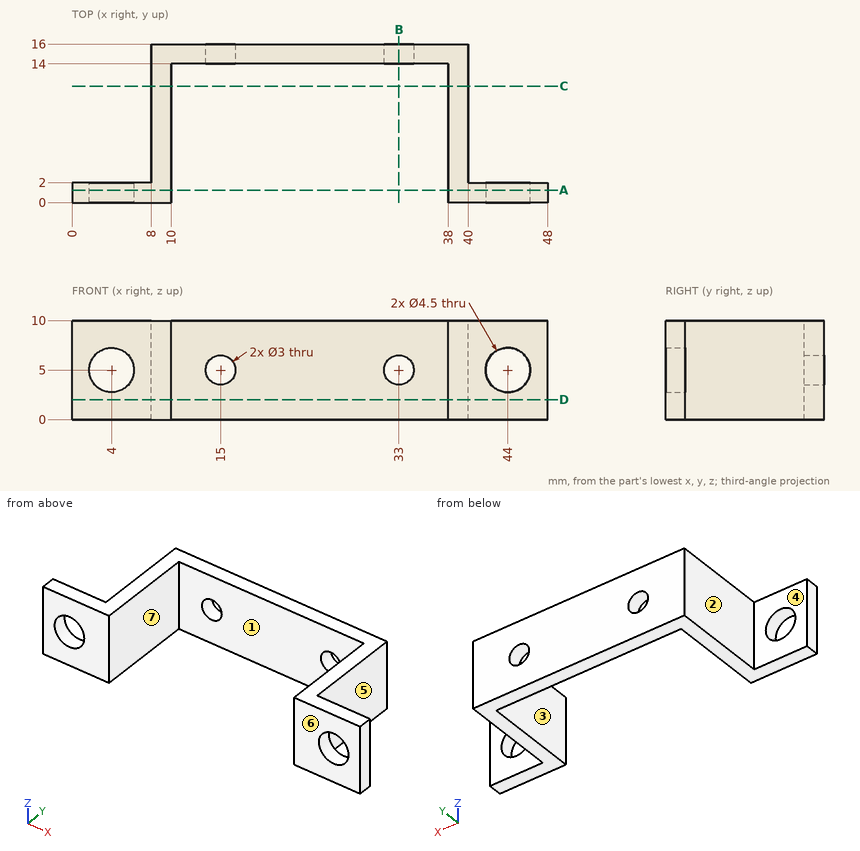
The drawing under review shows one solid part. Ordinate dimensions are in mm from its lowest x, y, z. A direction names the side the tool comes from. Coordinates: 2 decimals unless noted, no trailing zeros. Order: outer loops, then holes, each group sorted by start corner. A loop starts at its lowest first (then second) coordinate and runs counter-clockwise, first axis right, second up. Notation, with made-up numbers: (83, -27) -> (136, -27) arc R16 cw to (136, -23) -> close; hole circle Ø11 at (86, -18). An arc over 180 degrees is marked (long way). Return JSON: item names as keys, results as strings.
1. For line 1 (X direction, y = 0.7, z = 5); line 2 (X direction, y = 14.7, z = 5); line 3 (Z direction, x = 15, y = 14.45), list the stretches that pass through material, from the lowest coordinate up. Write a range as from..to.
Answer block:
{"line 1": "0..1.75, 6.25..10, 38..41.75, 46.25..48", "line 2": "8..13.5, 16.5..31.5, 34.5..40", "line 3": "0..3.5, 6.5..10"}
2. Machinability: for the marked faces 5, 6 and 7, which of the approach directions +Z, -Z, +X, -X, +Y, -Y give a long, thin tool a straight path to every point of the face, cutting with its end or side? Answer none if there is none.
Answer block:
{"face 5": "+Z, -Z, +X, +Y", "face 6": "+Z, -Z, +X, -X, -Y", "face 7": "+Z, -Z, -Y"}
3. We need section B-B on x = 33. Write out the cut boundary in (y, z), and give its area (3 significant figures).
Answer block:
{"outline": "(14, 0) -> (16, 0) -> (16, 3.5) -> (14, 3.5) -> close; (14, 6.5) -> (16, 6.5) -> (16, 10) -> (14, 10) -> close", "area": "14.0 mm²"}
4. We need section D-D on z = 2. Write out the cut boundary in (x, y).
Answer block:
{"outline": "(0, 0) -> (10, 0) -> (10, 14) -> (38, 14) -> (38, 0) -> (48, 0) -> (48, 2) -> (40, 2) -> (40, 16) -> (8, 16) -> (8, 2) -> (0, 2) -> close"}
5. We need section C-C on y = 11.75. Write out the cut boundary in (x, z), and give its area (3 significant figures).
Answer block:
{"outline": "(8, 0) -> (10, 0) -> (10, 10) -> (8, 10) -> close; (38, 0) -> (40, 0) -> (40, 10) -> (38, 10) -> close", "area": "40.0 mm²"}
6. We need section A-A on y = 1.25. Write out the cut boundary in (x, z).
Answer block:
{"outline": "(0, 0) -> (10, 0) -> (10, 10) -> (0, 10) -> close; (38, 0) -> (48, 0) -> (48, 10) -> (38, 10) -> close; hole circle Ø4.5 at (4, 5); hole circle Ø4.5 at (44, 5)"}
7. The part is to be moulded in two halves that separate along X. For the marked faces 1, 2, 3 and 4, say which applies: +X half, -X half, draft (parallel to the pull), parting line (faces both ways), or undercut.
Answer block:
{"face 1": "undercut", "face 2": "-X half", "face 3": "undercut", "face 4": "draft"}
8. For pin 1 Ø2.5 at (x, z) = (33, 5) entering from +Y; pin 2 Ø2.5 at (x, z) = (44.5, 7.5) entering from +Y; pin 3 Ø3 at (y, z) = (7, 4.5) entering from -X; pin 4 Ø3 at (y, z) = (5, 6.5) entering from +X, all flat-tipped, find the tip position at first contact; note any pin that passes through.
Answer block:
{"pin 1": "through", "pin 2": "y = 2", "pin 3": "x = 8", "pin 4": "x = 40"}
